The drawing under review shows one solid part. Ordinate dimensions are in mm from its lowest x, y, z. Round coordinates to 2 decimals unless told otherwise and drop trailing zeros. Order: outer loops, then holes, each group sorted by start corner. A loop starts at its lowest first (then second) coordinate and runs counter-clockwise, first axis right, second up.
1) Consider section A-A (y = 2.25). Give the boundary of the cut face in (x, z).
2) Mouldability with a two-part tool opening along Y and no side actions: class the marked faces 1, 2, 3 and 4 as pulls with the +Y half, pulls with the -Y half, needs draft (parallel to the pull), parting line crosses it, or undercut.
3) To check wall thickness, follow L1, parallel to Y at x = 9, z = 21; L2, parallel to Y at x = 44, z = 20.5; L3, parallel to X at y = 20, z = 2.75. State the ranges of each line that lie inside material, in increasing order.
4) Clearance check with flat-ended pins moving along their axes: P1, Ø12, axis at x = 18.5, y = 20.5, coming from the -Z side; P2, Ø5, axis at x = 44, y = 2.25, coming from the -Z side; P3, Ø5.5, axis at y = 17.5, z = 13, coming from the -X side (3 decimals); P4, Ø13, axis at y = 22.5, z = 9.5, coming from the +X side. State where each tip first meets the part, or that it passes through.
5) Consider section D-D (z = 16). Give the boundary of the cut face in (x, y), then the cut area to 3 significant figures.
6) Consider section B-B (x = 44). Give the boundary of the cut face in (y, z), then the cut area to 3 significant figures.
7) Consider section C-C (y = 17.5). Give the boundary of the cut face in (x, z), then the cut area to 3 significant figures.
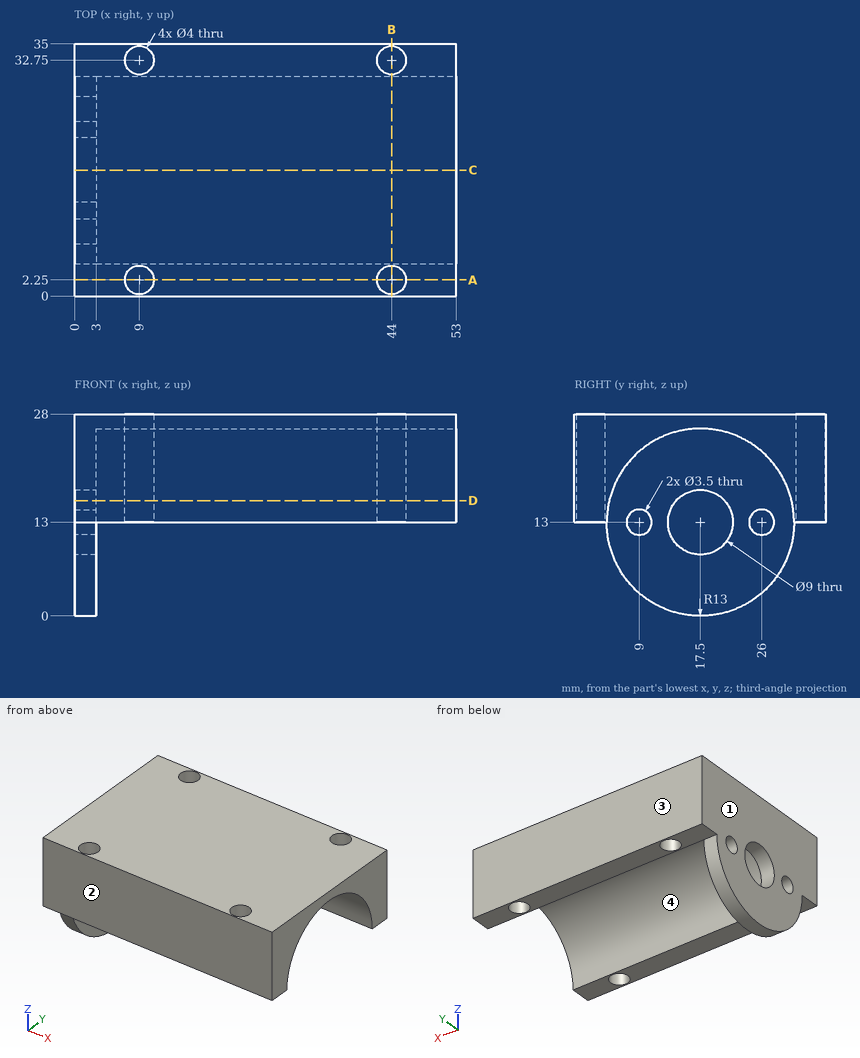
Answer below:
1. outline: (0, 13) - (7, 13) - (7, 28) - (0, 28) - close; (11, 13) - (42, 13) - (42, 28) - (11, 28) - close; (46, 13) - (53, 13) - (53, 28) - (46, 28) - close
2. face 1: needs draft
2. face 2: pulls with the -Y half
2. face 3: pulls with the +Y half
2. face 4: undercut
3. L1: y = 0 to 0.25, 4.25 to 7.25, 27.75 to 30.75, 34.75 to 35
3. L2: y = 0 to 0.25, 4.25 to 6.88, 28.12 to 30.75, 34.75 to 35
3. L3: x = 0 to 3
4. P1: stops at z = 22.38
4. P2: stops at z = 13
4. P3: passes through
4. P4: stops at x = 3
5. outline: (0, 0) - (53, 0) - (53, 4.85) - (3, 4.85) - (3, 14.15) - (0, 14.15) - close; (0, 20.85) - (3, 20.85) - (3, 30.15) - (53, 30.15) - (53, 35) - (0, 35) - close; hole circle Ø4 at (9, 2.25); hole circle Ø4 at (9, 32.75); hole circle Ø4 at (44, 2.25); hole circle Ø4 at (44, 32.75)
5. area: 520 mm2
6. outline: (0, 13) - (0.25, 13) - (0.25, 28) - (0, 28) - close; (4.25, 13) - (4.5, 13) arc R13 cw to (30.5, 13) - (30.75, 13) - (30.75, 28) - (4.25, 28) - close; (34.75, 13) - (35, 13) - (35, 28) - (34.75, 28) - close
6. area: 140 mm2
7. outline: (0, 0) - (3, 0) - (3, 8.5) - (0, 8.5) - close; (0, 17.5) - (3, 17.5) - (3, 26) - (53, 26) - (53, 28) - (0, 28) - close
7. area: 157 mm2
